Check sheet for the modelled part. Datum: model origin and axes. Units: mm. A direction names the side the tool comes from. Coordinates: 2 decimals unless noted, no trailing zeros. Loops run counter-clockwise (first coordinate to the right, second up) from the corner with the lowest first, then second, coordinate; pieces in that order, holes last. Notation, with made-up numbers: M 63.5,54.5 L 74.5,54.5 A19 ccw 74.5,88.5 Z; hole C -3.75,84 d11. An arc over 180 degrees is marked long. Use CSV: the item, a comma, the result in double quotes. Start each with the question number.
(1) Section check D-D on y = -1.3. Give the number of separate pieces and of enclosed holes in the cut face, and give its area (3 significant figures).
(2) Go/stop test with flat-tipped pins: pin 1 Ø13 at (x, z) = (10.31, -25.82) entering from -Y; pin 2 Ø22 at (x, z) = (-25.84, -45.59) entering from +Y; pin 3 Ø1.5 at (y, z) = (-1.5, -50.5) entering from +X; pin 4 Ø1 at (x, y) = (-46, -1.5) entering from +Z. Record where each tip stops, or that it passes through.
(3) Section check C-C on z = 57. Record the cut outline in (x, y) (3 decimals), and give its area (3 significant figures).
(4) Draft check along X on faces 3 (the cylindrical face through (-4.31, -1.57, -42.24)), 4 (the flat face through (62.893, -1.565, -17.551)), 5 (the flat face through (11, -3.175, 1)), 6 (the flat face through (-72.11, -1.57, 15.57)). Enter one of: pulls with the +X half, pulls with the -X half, needs draft (parallel to the pull), parting line crosses it, or undercut.
(5) Scan lines: line 1 (X direction, y = -0.5, z = -20.5); line 2 (Z direction, x = 19, y = -1.55) (3 decimals); line 3 (X direction, y = -2.55, z = 34.5). Record each from-to range of solid material in increasing order.
(6) Section check B-B on x = -42. Record the cut outline in (y, z) (3 decimals), and give its area (3 significant figures).
(7) Set-up check for faces 1 (the flat face through (47.36, -1.57, -45.95)), 2 (the flat face through (-60.59, -1.57, -9.43)): record each of +Z, -Z, +X, -X, +Y, -Y from which the full face is reachable in a straight line by a thin tool's end or side.
(8) Section check A-A on z = 0. Record the cut outline in (x, y) (3 decimals).
from build123d import *

# Parameters (mm, degrees)
F0_R     = 9.4996
F0_R_2   = 9.7028
F0_R_3   = 11.1633
F0_R_4   = 9.2583
F0_R_5   = 9.0932
F0_R_6   = 8.8773
F0_R_7   = 10.9474
F0_R_8   = 10.7442
F0_R_9   = 8.6741
F0_R_10  = 7.0231
F0_R_11  = 9.9187
F0_R_12  = 7.2263
F0_R_13  = 10.1219
F0_R_14  = 10.3378
F0_R_15  = 7.4295
F0_R_16  = 7.6327
F0_R_17  = 11.303
F0_R_18  = 10.541
F0_R_19  = 8.4582
F0_R_20  = 8.255
F0_R_21  = 8.0518
F0_R_22  = 7.8486
F1_DEPTH = 3.175


with BuildPart() as f1:
    # F0 (on Front) → F1 (new body)
    with BuildSketch(Plane.XZ):
        Polygon((-74.326232, 6.558197), (-58.00814, -3.154771), (-63.250169, -15.885411), (-61.209839, -38.620494), (-5.588048, -68.933934), (36.725905, -59.315246), (58.295086, -32.208033), (67.622297, -2.477541), (55.380326, 30.750657), (29.439015, 59.315246), (-5.588048, 68.64246), (-54.505903, 50.862461), (-69.954097, 24.338197), align=None)
        with Locations((-25.844501, -45.592066)):
            Circle(F0_R, mode=Mode.SUBTRACT)
        with Locations((-48.288107, -29.26944)):
            Circle(F0_R_2, mode=Mode.SUBTRACT)
        with Locations((-17.783852, -18.508689)):
            Circle(F0_R_3, mode=Mode.SUBTRACT)
        with Locations((-3.109419, -51.421572)):
            Circle(F0_R_4, mode=Mode.SUBTRACT)
        with Locations((21.957465, -49.672719)):
            Circle(F0_R_5, mode=Mode.SUBTRACT)
        with Locations((40.611893, -35.973374)):
            Circle(F0_R_6, mode=Mode.SUBTRACT)
        with Locations((10.305857, -25.8201)):
            Circle(F0_R_7, mode=Mode.SUBTRACT)
        with Locations((28.269259, -5.10082)):
            Circle(F0_R_8, mode=Mode.SUBTRACT)
        with Locations((52.270912, -13.821245)):
            Circle(F0_R_9, mode=Mode.SUBTRACT)
        with Locations((-63.44483, 12.994493)):
            Circle(F0_R_10, mode=Mode.SUBTRACT)
        with Locations((-43.915976, 0)):
            Circle(F0_R_11, mode=Mode.SUBTRACT)
        with Locations((-54.992042, 31.065969)):
            Circle(F0_R_12, mode=Mode.SUBTRACT)
        with Locations((-30.216632, 22.613181)):
            Circle(F0_R_13, mode=Mode.SUBTRACT)
        with Locations((-3.983845, 33.980723)):
            Circle(F0_R_14, mode=Mode.SUBTRACT)
        with Locations((-40.418271, 45.348264)):
            Circle(F0_R_15, mode=Mode.SUBTRACT)
        with Locations((-18.557616, 54.092523)):
            Circle(F0_R_16, mode=Mode.SUBTRACT)
        with Locations((-2.918608, 2.477541)):
            Circle(F0_R_17, mode=Mode.SUBTRACT)
        with Locations((18.168284, 21.44728)):
            Circle(F0_R_18, mode=Mode.SUBTRACT)
        with Locations((51.68796, 10.66269)):
            Circle(F0_R_19, mode=Mode.SUBTRACT)
        with Locations((41.194841, 32.523345)):
            Circle(F0_R_20, mode=Mode.SUBTRACT)
        with Locations((22.831891, 46.805643)):
            Circle(F0_R_21, mode=Mode.SUBTRACT)
        with Locations((4.177465, 55.258427)):
            Circle(F0_R_22, mode=Mode.SUBTRACT)
    extrude(amount=F1_DEPTH)


solid = f1.part
Outcome:
1,separate pieces,"1"
1,enclosed holes,"22"
1,area,"8,030 mm²"
2,pin 1,"passes through"
2,pin 2,"stops at y = 0"
2,pin 3,"stops at x = 44.34"
2,pin 4,"stops at z = 54.14"
3,outline,"M -37.62,-3.175 L -25.615,-3.175 L -25.615,0 L -37.62,0 Z; M -11.5,-3.175 L -3.475,-3.175 L -3.475,0 L -11.5,0 Z; M 11.83,-3.175 L 31.542,-3.175 L 31.542,0 L 11.83,0 Z"
3,area,"126 mm²"
4,face 3,"undercut"
4,face 4,"pulls with the +X half"
4,face 5,"needs draft"
4,face 6,"pulls with the -X half"
5,line 1,"x = -62.84 to -52.44, -44.14 to -28.77, -6.8 to 0.74, 19.87 to 46.74, 57.81 to 61.97"
5,line 2,"z = -63.345 to -58.272, -41.074 to -32.473, -19.167 to -10.534, 0.332 to 10.939, 31.955 to 39.724, 53.887 to 62.095"
5,line 3,"x = -64.04 to -61.35, -48.63 to -14.31, 6.34 to 33.18, 49.21 to 51.98"
6,outline,"M -3.175,-49.09 L 0,-49.09 L 0,-36.659 L -3.175,-36.659 Z; M -3.175,-21.88 L 0,-21.88 L 0,-9.732 L -3.175,-9.732 Z; M -3.175,9.732 L 0,9.732 L 0,38.089 L -3.175,38.089 Z; M -3.175,52.607 L 0,52.607 L 0,55.408 L -3.175,55.408 Z"
6,area,"177 mm²"
7,face 1,"-Z, +X, +Y, -Y"
7,face 2,"-X, +Y, -Y"
8,outline,"M -63.308,-3.175 L -53.835,-3.175 L -53.835,0 L -63.308,0 Z; M -33.997,-3.175 L -13.947,-3.175 L -13.947,0 L -33.997,0 Z; M 8.11,-3.175 L 18.813,-3.175 L 18.813,0 L 8.11,0 Z; M 37.725,-3.175 L 66.71,-3.175 L 66.71,0 L 37.725,0 Z"
